Design review of the part built by this model. Coordinates are the model's own, in mm. A direction names the side the tool comes from. Round coordinates to 2 decimals unless told otherwise and drop trailing zeros. Loops run counter-clockwise (first coordinate to the right, second up) from the corner with the lowest first, then second, coordinate; pieces in that order, holes last. Notation, with made-up numbers: (73.5, 63.25) - (107.5, 63.25) arc R3 ccw to (107.5, 68.25) - close; hole circle Ø5 at (38.25, 64.25). An arc over 180 degrees is marked (long way). Return JSON: item names as keys, results as strings. Group by question number.
(1) Clearance check with flat-ended pins moving along their axes: pin 1 (7.5 mm diameter, centred on x = 6.5, y = -10.5, fed in from +Z); pin 2 (7.5 mm diameter, centred on x = 3, y = -9.5, fed in from -Z); pin 3 (1.5 mm diameter, centred on y = -8, z = 0.5, fed in from +X). State where each tip first meets the part, or that it passes through.
(2) Wall thickness on L1, parallel to Z at x = 9, y = -10; L2, parallel to X at y = -16.5, z = 1; L3, parallel to Z at x = 12, y = 18.5: over which ranges is each line inside the solid? List them lowest first. Write a range as [from, to].
(3) We need section C-C, the plane y = 11.5. Write out the cut boundary in (x, z).
(4) The part is to be moulded in two halves that separate along X. For faces 1 (the flat face through (-12.5, 0, 0)), 2 (the flat face through (0, -12, 7.5)), 3 (the flat face through (12.5, 0, 0)), 4 (the flat face through (22.5, 12, 0)), say which applies: pulls with the +X half, pulls with the -X half, needs draft (parallel to the pull), parting line crosses it, or undercut.
(5) We need section A-A, the plane x = 3. Write out the cut boundary in (y, z).
(6) For faces 5 (the flat face through (0, 0, 2.5)), 6 (the flat face through (0, -12, -7.5)), 7 (the flat face through (-17.5, -12, 0)), list the 3-axis set-ups (+Z, -Z, +X, -X, +Y, -Y) from which the entire face can be reached by the end or side of a thin tool; tool diameter is ignored.
(7) We need section D-D, the plane x = 14. Write out the cut boundary in (y, z), and give its area (3 significant figures).
(8) We need section B-B, the plane z = -1.5. Write out the cut boundary in (x, y).
from build123d import *

# Parameters (mm, degrees)
SKETCH1_W           = 45
SKETCH1_H           = 25
SKETCH1_W_2         = 35
SKETCH1_H_2         = 15
SKETCH1_W_3         = 25
SKETCH1_H_3         = 5
BOSS_EXTRUDE1_DEPTH = 25
SKETCH1_3_W         = 35
SKETCH1_3_H         = 15
SKETCH1_3_W_2       = 25
SKETCH1_3_H_2       = 5
BOSS_EXTRUDE2_DEPTH = 25


with BuildPart() as part:
    # Sketch1 → Boss-Extrude1 (new body)
    # profile 1 of 2: a face of its own
    with BuildSketch(Plane(origin=(0, 0, 0), x_dir=(1, 0, 0), z_dir=(0, 1, 0))):
        Rectangle(SKETCH1_W, SKETCH1_H)
        Rectangle(SKETCH1_W_2, SKETCH1_H_2, mode=Mode.SUBTRACT)
    # profile 2 of 2: a face of its own
    with BuildSketch(Plane(origin=(0, 0, 0), x_dir=(1, 0, 0), z_dir=(0, 1, 0))):
        Rectangle(SKETCH1_W_2, SKETCH1_H_2)
        Rectangle(SKETCH1_W_3, SKETCH1_H_3, mode=Mode.SUBTRACT)
    extrude(amount=BOSS_EXTRUDE1_DEPTH)

    # Sketch1_3 → Boss-Extrude2 (add)
    with BuildSketch(Plane(origin=(0, 0, 0), x_dir=(1, 0, 0), z_dir=(0, 1, 0))):
        Rectangle(SKETCH1_3_W, SKETCH1_3_H)
        Rectangle(SKETCH1_3_W_2, SKETCH1_3_H_2, mode=Mode.SUBTRACT)
    extrude(amount=-BOSS_EXTRUDE2_DEPTH)


solid = part.part
Solutions:
{
 "1": {"pin 1": "z = 7.5", "pin 2": "z = -7.5", "pin 3": "x = 17.5"},
 "2": {"L1": "[-7.5, -2.5], [2.5, 7.5]", "L2": "[-17.5, -12.5], [12.5, 17.5]", "L3": "[-12.5, -2.5], [2.5, 12.5]"},
 "3": {"outline": "(-22.5, -12.5) - (22.5, -12.5) - (22.5, 12.5) - (-22.5, 12.5) - close; hole (-12.5, -2.5) - (12.5, -2.5) - (12.5, 2.5) - (-12.5, 2.5) - close"},
 "4": {"face 1": "undercut", "face 2": "needs draft", "face 3": "undercut", "face 4": "pulls with the +X half"},
 "5": {"outline": "(-25, -7.5) - (0, -7.5) - (0, -12.5) - (25, -12.5) - (25, -2.5) - (-25, -2.5) - close; (-25, 2.5) - (25, 2.5) - (25, 12.5) - (0, 12.5) - (0, 7.5) - (-25, 7.5) - close"},
 "6": {"face 5": "+Y, -Y", "face 6": "-Z, +X, -X, -Y", "face 7": "+Z, -Z, -X, -Y"},
 "7": {"outline": "(-25, -7.5) - (0, -7.5) - (0, -12.5) - (25, -12.5) - (25, 12.5) - (0, 12.5) - (0, 7.5) - (-25, 7.5) - close", "area": "1,000 mm^2"},
 "8": {"outline": "(-22.5, 0) - (-17.5, 0) - (-17.5, -25) - (-12.5, -25) - (-12.5, 25) - (-22.5, 25) - close; (12.5, -25) - (17.5, -25) - (17.5, 0) - (22.5, 0) - (22.5, 25) - (12.5, 25) - close"}
}
